For this review, take the finished solid that the model builds, in its own axes (mm). Face numbers are marked on the shaded views. Give positions to 0.01 mm unless a question says otherwise; leave off trailing zeros. Write each loop counter-clockwise with the first axis right and the second up, starting at its lowest first coordinate (ties: lowest second). Pieces come first, ordered by that corner, then holes. Notation, with made-up numbers: (7, 33) -> (62, 33) arc R21 cw to (62, 54) -> close; hole circle Ø7 at (-19.75, 51). An arc over 180 degrees is marked (long way). Write item = value, one per line.
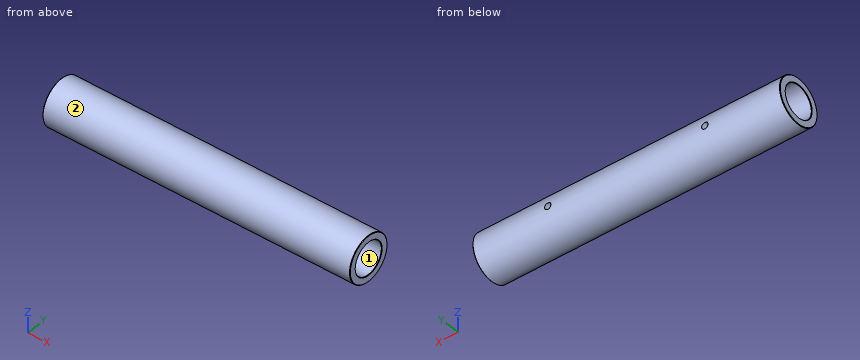
```python
from build123d import *

# Parameters (mm, degrees)
SKETCH_1_R              = 50
SKETCH_1_R_2            = 35
EXTRUDE_1_DEPTH         = 337.5
CHAMFER_1_SIZE          = 1
HOLE_WIZARD_M16_1_D     = 14
HOLE_WIZARD_M16_1_DEPTH = 42
HOLE_WIZARD_M16_1_TIP   = 4.206024333


with BuildPart() as part:
    # 草图1 → 凸台-拉伸1 (new, symmetric)
    with BuildSketch(Plane(origin=(0, 0, 0), x_dir=(0, 0, -1), z_dir=(1, 0, 0))):
        Circle(SKETCH_1_R)
        Circle(SKETCH_1_R_2, mode=Mode.SUBTRACT)
    extrude(amount=EXTRUDE_1_DEPTH, both=True)

    # 倒角1
    chamfer_1_edges = [part.edges().sort_by_distance(p)[0] for p in [
        (-337.5, 0, 50),
        (337.5, 0, 50),
        (-337.5, 0, 35),
        (337.5, 0, 35),
    ]]
    chamfer(chamfer_1_edges, length=CHAMFER_1_SIZE)

    # M16 螺纹孔1
    with Locations(Plane(origin=(0, 50, 0), x_dir=(1, 0, 0), z_dir=(0, 1, 0))):
        with Locations((172.5, 0), (-172.5, 0)):
            Hole(HOLE_WIZARD_M16_1_D / 2, depth=HOLE_WIZARD_M16_1_DEPTH)
            with Locations((0, 0, -(HOLE_WIZARD_M16_1_DEPTH + HOLE_WIZARD_M16_1_TIP / 2))):  # 118° drill point
                Cone(0, HOLE_WIZARD_M16_1_D / 2, HOLE_WIZARD_M16_1_TIP, mode=Mode.SUBTRACT)


solid = part.part
```
(1) Take a section at A-A (y = 0). Write out the cut boundary in (x, z), plus the area to 3 significant figures.
Answers below:
outline = (-337.5, -49) -> (-336.5, -50) -> (336.5, -50) -> (337.5, -49) -> (337.5, -36) -> (336.5, -35) -> (-336.5, -35) -> (-337.5, -36) -> close; (-337.5, 36) -> (-336.5, 35) -> (336.5, 35) -> (337.5, 36) -> (337.5, 49) -> (336.5, 50) -> (-336.5, 50) -> (-337.5, 49) -> close
area = 20,200 mm^2
(2) To check wall thickness, follow probe 1 along Z at (x, y) = (-6, 2); probe 2 along Z at (x, y) = (193, 1.5); probe 3 along Y at (x, z) = (75, 0). State the ranges of each line that lie inside material, in increasing order.
Answers below:
probe_1 = -49.96 to -34.94, 34.94 to 49.96
probe_2 = -49.98 to -34.97, 34.97 to 49.98
probe_3 = -50 to -35, 35 to 50
(3) Take a section at D-D (x = -172.5). Write out the cut boundary in (y, z), plus the area to 3 significant figures.
Answers below:
outline = (34.29, -7) arc R35 cw (long way) to (34.29, 7) -> (49.51, 7) arc R50 ccw (long way) to (49.51, -7) -> close
area = 3,790 mm^2
(4) Take a section at B-B (z = 0). Write out the cut boundary in (x, y).
Answers below:
outline = (-337.5, -49) -> (-336.5, -50) -> (336.5, -50) -> (337.5, -49) -> (337.5, -36) -> (336.5, -35) -> (-336.5, -35) -> (-337.5, -36) -> close; (-337.5, 36) -> (-336.5, 35) -> (-179.5, 35) -> (-179.5, 50) -> (-336.5, 50) -> (-337.5, 49) -> close; (-165.5, 35) -> (165.5, 35) -> (165.5, 50) -> (-165.5, 50) -> close; (179.5, 35) -> (336.5, 35) -> (337.5, 36) -> (337.5, 49) -> (336.5, 50) -> (179.5, 50) -> close
(5) Take a section at C-C (x = -90). Write out the cut boundary in (y, z), plus the area to 3 significant figures.
Answers below:
outline = circle Ø100 at (0, 0); hole circle Ø70 at (0, 0)
area = 4,010 mm^2
(6) The part is to be moulded in two halves that separate along Z. For the marked faces 1 and 2, say which applies: released by +Z, released by -Z, zero draft, split by the parting line, or undercut.
Answers below:
face_1 = undercut
face_2 = split by the parting line
(7) For pin 1 (10 mm diameter, centred on x = -192, y = -34.5, fed in from +Z); pin 2 (5 mm diameter, centred on x = 6, y = -24, fed in from +Z); pin 3 (8 mm diameter, centred on x = -177.5, y = -16.5, fed in from +Z), all flat-tipped, find the tip position at first contact; note any pin that passes through.
Answers below:
pin_1 = 40.37
pin_2 = 45.14
pin_3 = 48.41
